Geometry: final body of the model. Coordinates: model frame, mm. A direction names the side the tool comes from. Round coordinates to 2 decimals unless told otherwise and drop trailing zeros. Loops run counter-clockwise (first coordinate to the right, second up) from the corner with the lowest first, then second, coordinate; pieces in that order, holes last. Notation, with made-up numbers: (82, -22.75) -> (97, -22.75) arc R16 cw to (97, -8.75) -> close; hole circle Ø5 at (70.5, -1.75). An arc over 180 degrees is marked (long way). Answer in a Markdown table with one row per item.
```python
from build123d import *

# Parameters (mm, degrees)
SKETCH1_R               = 26
BOSS_EXTRUDE1_DEPTH     = 33
SHELL1_START            = 2
SHELL1_OUTLINE_R        = 28
SHELL1_DEPTH            = 29
SKETCH2_W               = 29
SKETCH2_H               = 54
CUT_EXTRUDE1_DEPTH      = 53
SKETCH3_R               = 26
BOSS_EXTRUDE2_DEPTH     = 2
SKETCH4_R               = 31.708367963
CUT_EXTRUDE2_DEPTH      = 29
SKETCH5_R               = 2.25
BOSS_EXTRUDE3_DEPTH     = 4
FILLET1_R               = 2
CHAMFER1_SIZE           = 3.326511139
BOSS_EXTRUDE4_START     = -33
BOSS_EXTRUDE4_OUTLINE_R = 2.25
BOSS_EXTRUDE4_DEPTH     = 33
FILLET2_R               = 4.75


with BuildPart() as part:
    # Sketch1 → Boss-Extrude1 (new body)
    with BuildSketch(Plane(origin=(0, 0, 0), x_dir=(0, 0, -1), z_dir=(1, 0, 0))):
        with BuildLine():
            Line((52, 0), (52, 50))
            Line((52, 50), (0, 50))
            Line((0, 50), (-6, 50))
            Line((-6, 50), (-6, 40))
            ThreePointArc((-6, 40), (-32.429333818, 27.334633781), (-43, 0))
            ThreePointArc((-43, 0), (4.5, -47.1), (52, 0))
        make_face()
        Circle(SKETCH1_R, mode=Mode.SUBTRACT)
    extrude(amount=BOSS_EXTRUDE1_DEPTH)

    # Shell1: read off the stored shape, not the designer's step
    # Shell1 outline → Shell1 (cut)
    with BuildSketch(Plane.YZ.offset(SHELL1_START)):
        with BuildLine():
            ThreePointArc((0.016913017, 41.000071514), (-45.099999808, -4.495817139), (0.0085476, -50))
            Line((0.0085476, -50), (48, -50))
            Line((48, -50), (48, 4))
            Line((48, 4), (38.088170021, 4))
            ThreePointArc((38.088170021, 4), (26.652605024, 30.320127965), (0.016913017, 41.000071514))
        make_face()
        Circle(SHELL1_OUTLINE_R, mode=Mode.SUBTRACT)
    extrude(amount=SHELL1_DEPTH, mode=Mode.SUBTRACT)

    # Sketch2 → Cut-Extrude1 (cut)
    with BuildSketch(Plane(origin=(0, 50, 0), x_dir=(1, 0, 0), z_dir=(0, 1, 0))):
        with Locations((16.5, 23)):
            Rectangle(SKETCH2_W, SKETCH2_H)
    extrude(amount=-CUT_EXTRUDE1_DEPTH, mode=Mode.SUBTRACT)

    # Sketch3 → Boss-Extrude2 (add)
    with BuildSketch(Plane.ZY):
        with Locations(Location((0, 0, 0), (0, 0, 81.150116902))):
            Circle(SKETCH3_R)
    extrude(amount=-BOSS_EXTRUDE2_DEPTH)

    # Sketch4 → Cut-Extrude2 (cut)
    with BuildSketch(Plane(origin=(31, 0, 0), x_dir=(0, 0, -1), z_dir=(1, 0, 0))):
        Circle(SKETCH4_R)
    extrude(amount=-CUT_EXTRUDE2_DEPTH, mode=Mode.SUBTRACT)

    # Sketch5 → Boss-Extrude3 (add)
    # profile 1 of 2: a face of its own
    with BuildSketch(Plane.ZY):
        with BuildLine():
            ThreePointArc((-51.418984108, -30.13414218), (-48.82497471, -34.177482297), (-45.913745602, -37.998768617))
            Line((-45.913745602, -37.998768617), (-38.477731669, -32.793558864))
            ThreePointArc((-38.477731669, -32.793558864), (-41.663875667, -29.183056126), (-44.468117742, -25.268535724))
            Line((-44.468117742, -25.268535724), (-51.418984108, -30.13414218))
        make_face()
        with Locations((-45, -31.5)):
            Circle(SKETCH5_R, mode=Mode.SUBTRACT)
    # profile 2 of 2: a face of its own
    with BuildSketch(Plane.ZY):
        with BuildLine():
            ThreePointArc((32.398527193, 27.367900169), (35.450790949, 23.647327492), (38.031195395, 19.585248223))
            Line((38.031195395, 19.585248223), (45.075911525, 24.281725643))
            ThreePointArc((45.075911525, 24.281725643), (42.60097507, 28.400650047), (39.750789641, 32.269408468))
            Line((39.750789641, 32.269408468), (32.398527193, 27.367900169))
        make_face()
        with Locations((39, 26)):
            Circle(SKETCH5_R, mode=Mode.SUBTRACT)
    extrude(amount=-BOSS_EXTRUDE3_DEPTH)

    # Fillet1
    fillet1_edges = [part.edges().sort_by_distance(p)[0] for p in [
        (2, -30.13414218, -51.418984108),
    ]]
    fillet(fillet1_edges, radius=FILLET1_R)

    # Chamfer1
    # the kernel refuses this chamfer: 3.326511139, 3 mm, written as the material it takes off along each edge
    with BuildSketch(Plane(origin=(-8.575137871, 24.281725643, 45.075911525), x_dir=(0, -0.5547001962252163, -0.8320502943378523), z_dir=(1, 0, 0))) as chamfer1_piece_1:
        with BuildLine():
            Line((CHAMFER1_SIZE, 0), (-0.190667191, 2.911795765))
            ThreePointArc((-0.190667191, 2.911795765), (-0.119044869, 1.500102705), (0, 0))
            Line((0, 0), (CHAMFER1_SIZE, 0))
        make_face()
    extrude(amount=21.150275743, mode=Mode.SUBTRACT)

    # Boss-Extrude4: read off the stored shape, not the designer's step
    # Boss-Extrude4 outline → Boss-Extrude4 (add)
    # profile 1 of 2: a face of its own
    with BuildSketch(Plane.ZY.offset(BOSS_EXTRUDE4_START)):
        with BuildLine():
            ThreePointArc((26.336648486, 32.700609517), (29.932721568, 29.805201706), (33.168906621, 26.512446886))
            Line((33.168906621, 26.512446886), (39.750789641, 32.269408468))
            ThreePointArc((39.750789641, 32.269408468), (36.48342014, 35.922138784), (32.881782461, 39.245743491))
            Line((32.881782461, 39.245743491), (26.336648486, 32.700609517))
        make_face()
        with Locations((32, 32)):
            Circle(BOSS_EXTRUDE4_OUTLINE_R, mode=Mode.SUBTRACT)
    # profile 2 of 2: a face of its own
    with BuildSketch(Plane.ZY.offset(BOSS_EXTRUDE4_START)):
        with BuildLine():
            Line((-38.840294261, -45.204092661), (-31.980263742, -38.344223418))
            ThreePointArc((-31.980263742, -38.344223418), (-35.639554577, -35.469452882), (-39, -32.250427936))
            Line((-39, -32.250427936), (-45.913745602, -37.998768617))
            ThreePointArc((-45.913745602, -37.998768617), (-42.529883516, -41.751496496), (-38.840294261, -45.204092661))
        make_face()
        with Locations((-39, -39)):
            Circle(BOSS_EXTRUDE4_OUTLINE_R, mode=Mode.SUBTRACT)
    extrude(amount=BOSS_EXTRUDE4_DEPTH)

    # Fillet2
    # the kernel refuses this fillet: 4.75 mm, written as the material it takes off along each edge
    with BuildSketch(Plane(origin=(45.884989722, -37.998768617, -45.913745602), x_dir=(0, -0.742095530004095, 0.6702941327118576), z_dir=(-1, 0, 0))) as fillet2_piece_1:
        with BuildLine():
            CenterArc((4.948609093, 4.745557529), FILLET2_R, 177.651602882, 94.826600607)
            Line((0.202598429, 4.940192516), (0, 0))
            ThreePointArc((0, 0), (2.576997944, -0.055739892), (5.153995889, 0))
        make_face()
    extrude(amount=41.884989722, mode=Mode.SUBTRACT)
    with BuildSketch(Plane(origin=(44.936529157, -45.204092661, -38.840294261), x_dir=(0, 0.6815583401392785, -0.7317637794989523), z_dir=(-1, 0, 0))) as fillet2_piece_2:
        with BuildLine():
            CenterArc((4.584343333, -4.746187729), FILLET2_R, 87.70431796, 90.260546116)
            Line((-0.162660545, -4.577504047), (0, 0))
            ThreePointArc((0, 0), (2.387305831, 0.047832742), (4.774611663, 0))
        make_face()
    extrude(amount=56.873058314, mode=Mode.SUBTRACT)
    with BuildSketch(Plane(origin=(44.949107529, 39.245743491, 32.881782461), x_dir=(0, -0.6773005061883329, 0.735706479730217), z_dir=(-1, 0, 0))) as fillet2_piece_3:
        with BuildLine():
            CenterArc((4.557931056, -4.744822843), FILLET2_R, 87.324678627, 90.308374896)
            Line((-0.188016347, -4.548651358), (0, 0))
            ThreePointArc((0, 0), (2.389821506, 0.055804306), (4.779643012, 0))
        make_face()
    extrude(amount=56.898215059, mode=Mode.SUBTRACT)
    with BuildSketch(Plane(origin=(45.609389119, 32.269408468, 39.750789641), x_dir=(0, -0.6583630051662173, -0.7527005735539911), z_dir=(-1, 0, 0))) as fillet2_piece_4:
        with BuildLine():
            CenterArc((4.804098652, -4.75), FILLET2_R, 90, 93.540841906)
            ThreePointArc((0.06316627, -5.043360096), (-0.030557791, -2.522458341), (0, 0))
            Line((0, 0), (4.804098652, 0))
        make_face()
    extrude(amount=41.609389119, mode=Mode.SUBTRACT)


solid = part.part
```
Item 1: Mould query, pull axis Y, two halves, no side actions, for faces 6 (the flat face through (4, 28.4, 39.5)), 7 (the flat face through (16, 24, -50)), 8 (the cylindrical face through (16.731, -43.356, -39.023)), 9 (the flat face through (16.731, 34.387, 28.023)). Classes: released by +Y, released by -Y, zero draft, split by the parting line, or undercut.
Ans:
| item | result |
|---|---|
| face 6 | undercut |
| face 7 | zero draft |
| face 8 | released by -Y |
| face 9 | released by +Y |
Item 2: Section query C-C, the plane y = 13.5. Output: boundary loops of the cut face in (x, z), and give its area (3 significant figures).
Ans:
| item | result |
|---|---|
| outline | (0, -52) -> (33, -52) -> (33, -22.22) -> (31, -22.22) -> (31, -50) -> (2, -50) -> (2, 38.63) -> (31, 38.63) -> (31, 22.22) -> (33, 22.22) -> (33, 40.76) -> (0, 40.76) -> close |
| area | 402 mm2 |
Item 3: Section query B-B, the plane z = -14. Output: boundary loops of the cut face in (x, y).
Ans:
| item | result |
|---|---|
| outline | (0, -46.14) -> (33, -46.14) -> (33, -21.91) -> (31, -21.91) -> (31, -44.1) -> (2, -44.1) -> (2, 50) -> (0, 50) -> close; (31, 21.91) -> (33, 21.91) -> (33, 50) -> (31, 50) -> close |
Item 4: Ray query, L1, parallel to X at y = 42.5, z = -16.5; L2, parallel to Z at x = 15, y = 33.5; L3, parallel to Z at x = 10.5, y = -39.5. Return the intervals inside material, ascending.
Ans:
| item | result |
|---|---|
| L1 | 0 to 2, 31 to 33 |
| L2 | -52 to -50, 21.3 to 25.17, 27.14 to 30.32, 33.68 to 37.69 |
| L3 | -43.72 to -41.19, -36.81 to -33.14, -30.27 to -26.37, 17.37 to 21.27 |
Item 5: Section query A-A, the plane z = 32. Output: boundary loops of the cut face in (x, y), and give its area (3 significant figures).
Ans:
| item | result |
|---|---|
| outline | (0, -30) -> (33, -30) -> (33, 29.75) -> (0, 29.75) -> close; (0, 34.25) -> (33, 34.25) -> (33, 37.31) -> (0, 37.31) -> close; hole (2, -26.77) -> (31, -26.77) -> (31, 24.81) -> (2, 24.81) -> close |
| area | 577 mm2 |
Item 6: First-contact query: P1, Ø2.5, axis at y = -39, z = -39, coming from the -X side; P2, Ø8, axis at x = 24, y = 4.5, coming from the +Z side; P3, Ø5, axis at x = 8, z = 31.5, coming from the +Y side; P4, Ø12, axis at x = 23.5, z = 26.5, coming from the -Y side. Flat tips, straight axial feed; report the tip coordinate or a pass-through.
Ans:
| item | result |
|---|---|
| P1 | through |
| P2 | z = 43 |
| P3 | y = 37.42 |
| P4 | y = -39.99 |
Item 7: Set-up query: faces 1 (the flat face through (4, -34, -46)), 2 (the flat face through (16.731, -40.18, -33.816)), 3 (the cylindrical face through (16.3, 26.95, 30.03)), 4 (the cylindrical face through (16.27, 14.35, 40.45)), 5 (the flat face through (1.97, 20.99, 40.14)). Return all of +Z, -Z, +X, -X, +Y, -Y with unobstructed straight access to the full face (end or side cutting, diameter ignored); none if empty.
Ans:
| item | result |
|---|---|
| face 1 | -Z, +X |
| face 2 | +X, -X, -Y |
| face 3 | none |
| face 4 | +Z, +X |
| face 5 | +Z, +X, -X |
Item 8: Section query D-D, the plane x = 29. Output: boundary loops of the cut face in (y, z), and give its area (3 significant figures).
Ans:
| item | result |
|---|---|
| outline | (-41.97, -35.6) arc R4.75 ccw to (-41.95, -42.33) arc R59.6 ccw to (-41.82, -42.46) arc R4.75 ccw to (-34.84, -42.11) -> (-32.25, -39) arc R47.5 ccw to (0, -52) -> (50, -52) -> (50, -50) -> (-3, -50) -> (-3, -49.87) arc R45.5 cw to (0.02, 41) arc R37.76 cw to (38.09, 4) -> (50, 4) -> (50, 6) -> (40, 6) arc R39.76 ccw to (32.7, 26.34) -> (36.03, 29.66) arc R4.75 ccw to (36.02, 36.39) arc R4.75 ccw to (29.11, 36.13) -> (26.51, 33.17) arc R39.76 ccw to (0, 43) arc R47.5 ccw to (-38.34, -31.98) -> close; hole circle Ø4.5 at (-39, -39); hole circle Ø4.5 at (32, 32) |
| area | 655 mm2 |
